Check sheet for the modelled part. Datum: model origin and axes. Units: mm. Round coordinates to 2 decimals unless told otherwise and drop trailing zeros. Loops run counter-clockwise (first coordinate to the right, second up) from the corner with the lowest first, then second, coordinate; pieces in that order, holes last. Notation, with made-up numbers: (-37.5, 53) -> (6.5, 53) arc R27 ccw to (6.5, 74) -> close; hole circle Ø11 at (7.25, 77.5). An arc over 180 degrees is marked (long way). Return JSON: item names as keys, results as strings.
from build123d import *

# Parameters (mm, degrees)
BOSS_EXTRUDE1_DEPTH = 400
BOSS_EXTRUDE3_DEPTH = 60
FILLET4_R           = 10
SKETCH6_R           = 1.25
SKETCH6_W           = 43.954521952
SKETCH6_H           = 12
CUT_EXTRUDE5_DEPTH  = 50
BOSS_EXTRUDE4_START = -10
BOSS_EXTRUDE4_DEPTH = 10
BOSS_EXTRUDE5_DEPTH = 7
SKETCH10_W          = 10
SKETCH10_H          = 5
BOSS_EXTRUDE6_DEPTH = 4
FILLET6_R           = 5
FILLET7_R           = 2


with BuildPart() as part:
    # Sketch1 → Boss-Extrude1 (new body)
    with BuildSketch(Plane.XY):
        with BuildLine():
            Line((-85, 0), (-82, 0))
            ThreePointArc((-82, 0), (0, 82), (82, 0))
            Line((82, 0), (85, 0))
            ThreePointArc((85, 0), (0, 85), (-85, 0))
        make_face()
    extrude(amount=BOSS_EXTRUDE1_DEPTH)

    # Sketch5 → Boss-Extrude3 (add)
    with BuildSketch(Plane(origin=(0, 0, 0), x_dir=(-1, 0, 0), z_dir=(0, 0, -1))):
        with BuildLine():
            Line((-21.977260976, 79), (21.977260976, 79))
            ThreePointArc((21.977260976, 79), (0, 82), (-21.977260976, 79))
        make_face()
    extrude(amount=-BOSS_EXTRUDE3_DEPTH)

    # Fillet4
    # the kernel refuses this fillet: 10 mm, written as the material it takes off along each edge
    with BuildSketch(Plane(origin=(46.977260976, 79, 60), x_dir=(0, 0, -1), z_dir=(-1, 0, 0))) as fillet4_piece_1_section:
        with BuildLine():
            CenterArc((FILLET4_R, -FILLET4_R), FILLET4_R, 90, 90)
            Line((0, -FILLET4_R), (0, 0))
            Line((0, 0), (FILLET4_R, 0))
        make_face()
    fillet4_piece_1 = extrude(amount=93.954521952, mode=Mode.PRIVATE)
    fillet4_piece_1 = fillet4_piece_1 & Plane(origin=(0, 0, 56.767461198), x_dir=(-1, 0, 0), z_dir=(0, 0, -1)) * Cylinder(82, 228, mode=Mode.PRIVATE)
    add(fillet4_piece_1, mode=Mode.SUBTRACT)

    # Sketch6 → Cut-Extrude5 (cut)
    with BuildSketch(Plane.XZ.offset(-79)):
        with Locations(Location((0, 37, 0), (0, 0, 270))):
            Circle(SKETCH6_R)
        with Locations(Location((10.392304845, 19, 0), (0, 0, 270))):
            Circle(SKETCH6_R)
        with Locations(Location((-10.392304845, 19, 0), (0, 0, 270))):
            Circle(SKETCH6_R)
        with Locations((0, 6)):
            Rectangle(SKETCH6_W, SKETCH6_H)
    extrude(amount=-CUT_EXTRUDE5_DEPTH, mode=Mode.SUBTRACT)

    # Sketch7 → Boss-Extrude4 (add)
    with BuildSketch(Plane.XY.offset(400).offset(BOSS_EXTRUDE4_START)):
        with BuildLine():
            Line((-75, 0), (-82, 0))
            ThreePointArc((-82, 0), (0, 82), (82, 0))
            Line((82, 0), (75, 0))
            ThreePointArc((75, 0), (0, 75), (-75, 0))
        make_face()
    extrude(amount=BOSS_EXTRUDE4_DEPTH)

    # Sketch9 → Boss-Extrude5 (add)
    with BuildSketch(Plane.XY.offset(400)):
        with BuildLine():
            Line((-5, 84.852813742), (-5, 80))
            Line((-5, 80), (-5, 74.833147735))
            Line((-5, 74.833147735), (-5, 70))
            Line((-5, 70), (5, 70))
            Line((5, 70), (5, 74.833147735))
            Line((5, 74.833147735), (5, 80))
            Line((5, 80), (5, 84.852813742))
            ThreePointArc((5, 84.852813742), (0, 85), (-5, 84.852813742))
        make_face()
    extrude(amount=BOSS_EXTRUDE5_DEPTH)

    # Sketch10 → Boss-Extrude6 (add)
    with BuildSketch(Plane.XY.offset(407)):
        with Locations((0, 72.5)):
            Rectangle(SKETCH10_W, SKETCH10_H)
    extrude(amount=BOSS_EXTRUDE6_DEPTH)

    # Fillet6
    fillet6_edges = [part.edges().sort_by_distance(p)[0] for p in [
        (80, 0, 400),
        (83.5, 0, 0),
        (-83.5, 0, 0),
        (-80, 0, 400),
    ]]
    fillet(fillet6_edges, radius=FILLET6_R)

    # Fillet7
    fillet7_edges = [part.edges().sort_by_distance(p)[0] for p in [
        (0, 79, 12),
    ]]
    fillet(fillet7_edges, radius=FILLET7_R)


solid = part.part
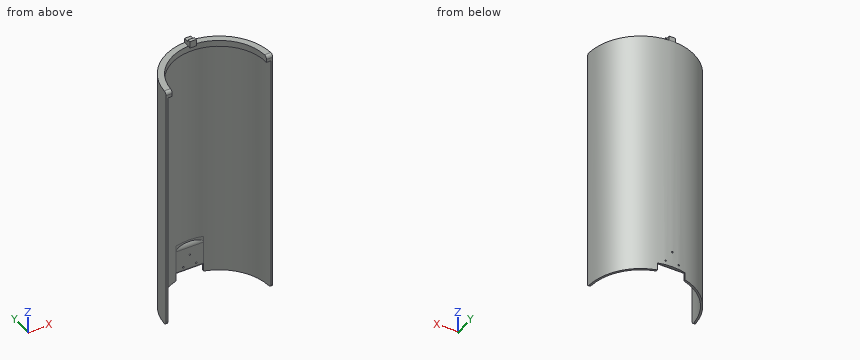
Q1. Section check C-C (z = 196). Record the boundary of the cut face in (x, y), then the cut area to 3 significant figures.
Results list:
{"outline": "(-85, 0) -> (-82, 0) arc R82 cw to (82, 0) -> (85, 0) arc R85 ccw to start", "area": "787 mm^2"}
Q2. Section check B-B (y = 44). Record the boundary of the cut face in (x, z).
Results list:
{"outline": "(-72.73, 0) -> (-69.2, 0) -> (-69.2, 390) -> (-60.74, 390) -> (-60.74, 400) -> (-72.73, 400) -> close; (60.74, 390) -> (69.2, 390) -> (69.2, 0) -> (72.73, 0) -> (72.73, 400) -> (60.74, 400) -> close"}
Q3. Section check A-A (y = 19). Record the boundary of the cut face in (x, z).
Results list:
{"outline": "(-82.85, 0) -> (-79.77, 0) -> (-79.77, 390) -> (-72.55, 390) -> (-72.55, 400) -> (-82.85, 400) -> close; (72.55, 390) -> (79.77, 390) -> (79.77, 0) -> (82.85, 0) -> (82.85, 400) -> (72.55, 400) -> close"}
Q4. Section check D-D (x = 62). Record the boundary of the cut face in (y, z).
Results list:
{"outline": "(42.2, 390) -> (53.67, 390) -> (53.67, 0) -> (58.15, 0) -> (58.15, 400) -> (42.2, 400) -> close"}
Q5. Material ranges on line 1 (X direction, y = 6, z = 319); line 2 (X direction, y = 28, z = 192.5); line 3 (Y direction, x = 22, z = 87.5), recorded low to high.
Results list:
{"line 1": "-84.79 to -81.78, 81.78 to 84.79", "line 2": "-80.26 to -77.07, 77.07 to 80.26", "line 3": "78.99 to 82.1"}
Q6. Go/stop test with flat-tipped pins: pin 1 (10 mm diameter, centred on x = -46.5, z = 95.5, fed in from +Y); pin 2 (2 mm diameter, centred on y = 59.5, z = 277.5, fed in from +X); pin 3 (8 mm diameter, centred on x = 40, z = 165, fed in from +Y). Record where each tip stops, or that it passes through.
Results list:
{"pin 1": "y = 74.18", "pin 2": "x = 61.67", "pin 3": "y = 77"}
